from build123d import *

# Parameters (mm, degrees)
F0_R      = 1.6
F1_DEPTH  = 4.75
F2_W      = 25
F2_H      = 11
F3_DEPTH  = 12
F5_DEPTH  = 6
F7_DEPTH  = 5.5
F8_W      = 12
F8_H      = 11
F9_DEPTH  = 2
F10_W     = 12
F10_H     = 11
F11_DEPTH = 2
F12_R     = 1.45
F14_DEPTH = 25
F13_R     = 1.45
F15_DEPTH = 25
F16_R     = 5


with BuildPart() as f1:
    # F0 (on Front) → F1 (new body, symmetric)
    with BuildSketch(Plane.XZ):
        with BuildLine():
            ThreePointArc((35.398387, -3.5), (40.348135, 8.449747), (28.398387, 3.5))
            Line((28.398387, 3.5), (-35.398387, 3.5))
            ThreePointArc((-35.398387, 3.5), (-38.898387, 0), (-35.398387, -3.5))
            Line((-35.398387, -3.5), (35.398387, -3.5))
        make_face()
        with Locations((35.398387, 3.5)):
            Circle(F0_R, mode=Mode.SUBTRACT)
    extrude(amount=F1_DEPTH, both=True)

    # F2 (on face) → F3 (join)
    with BuildSketch(Plane(origin=(0, 4.75, 0), x_dir=(-1, 0, 0), z_dir=(0, 1, 0))):
        with Locations((0, 2)):
            Rectangle(F2_W, F2_H)
    extrude(amount=-F3_DEPTH)

    # F4 (on face) → F5 (cut)
    with BuildSketch(Plane.XY.offset(7.5)):
        with BuildLine():
            Line((-6, -7.25), (6, -7.25))
            ThreePointArc((6, -7.25), (0, -1.25), (-6, -7.25))
        make_face()
        with BuildLine():
            ThreePointArc((-6, -7.25), (0, -13.25), (6, -7.25))
            Line((6, -7.25), (-6, -7.25))
        make_face()
    extrude(amount=-F5_DEPTH, mode=Mode.SUBTRACT)

    # F6 (on face) → F7 (cut)
    with BuildSketch(Plane(origin=(0, 0, -3.5), x_dir=(1, 0, 0), z_dir=(0, 0, -1))):
        with BuildLine():
            Line((-8, 7.25), (8, 7.25))
            ThreePointArc((8, 7.25), (0, 15.25), (-8, 7.25))
        make_face()
        with BuildLine():
            ThreePointArc((-8, 7.25), (0, -0.75), (8, 7.25))
            Line((8, 7.25), (-8, 7.25))
        make_face()
    extrude(amount=-F7_DEPTH, mode=Mode.SUBTRACT)

    # F8 (on face) → F9 (join)
    with BuildSketch(Plane.YZ.offset(12.5)):
        with Locations((-1.25, 2)):
            Rectangle(F8_W, F8_H)
    extrude(amount=F9_DEPTH)

    # F10 (on face) → F11 (join)
    with BuildSketch(Plane(origin=(-12.5, 0, 0), x_dir=(0, -1, 0), z_dir=(-1, 0, 0))):
        with Locations((1.25, 2)):
            Rectangle(F10_W, F10_H)
    extrude(amount=F11_DEPTH)

    # F12 (on face) → F14 (cut)
    with BuildSketch(Plane.XZ.offset(7.25)):
        with Locations((-12.05, 3.05)):
            Circle(F12_R)
    extrude(amount=-F14_DEPTH, mode=Mode.SUBTRACT)

    # F13 (on face) → F15 (cut)
    with BuildSketch(Plane.XZ.offset(7.25)):
        with Locations((12.05, 3.05)):
            Circle(F13_R)
    extrude(amount=-F15_DEPTH, mode=Mode.SUBTRACT)

    # F16
    f16_edges = [f1.edges().sort_by_distance(p)[0] for p in [
        (-14.5, -6, -3.5),
        (-14.5, -1.25, 7.5),
        (14.5, -6, -3.5),
        (14.5, -1.25, 7.5),
    ]]
    fillet(f16_edges, radius=F16_R)


solid = f1.part
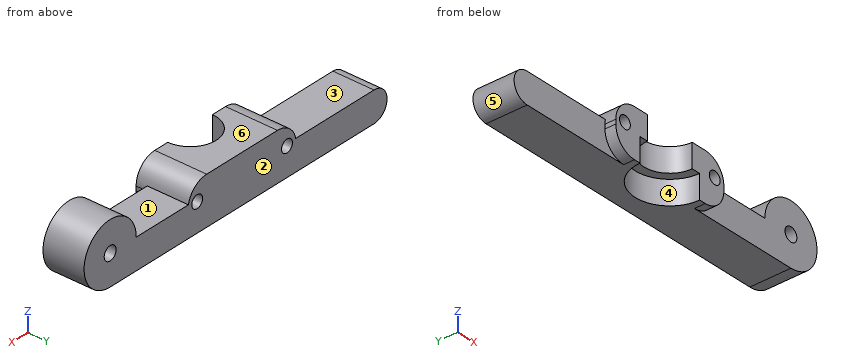
Check sheet for the modelled part. Datum: model origin and axes. Units: mm. Face numbers are marked on the shaded views. A direction names the side the tool comes from. Round coordinates to 2 decimals unless told otherwise and drop trailing zeros. Write each loop counter-clockwise with the first axis right and the second up, starting at its lowest first coordinate (ties: lowest second). Pieces come first, ordered by that corner, then holes. Notation, with made-up numbers: (-1.5, 80) -> (16.5, 80) arc R23 ccw to (16.5, 96) -> close; hole circle Ø6 at (88.25, 17). An arc over 180 degrees is marked (long way). Answer as CSV lines item,"result". Start each with the question number.
1) Material ranges on line 1 (X direction, y = -3, z = 3.75); line 2 (X direction, y = -3.75, z = 6.25); line 3 (Z direction, x = 9.5, y = 4), recorded low to high. Write a range as from..to.
2) Tool access check on the marked faces 1, 2 and 3. Record the directions out of +Z, -Z, +X, -X, +Y, -Y that give a thin tool (end or side, any length) a straight path to the whole face; none if there is none.
3) Section check D-D on x = 32. Enter the section's corners in (y, z).
4) Section check C-C on x = 0. Enter the section's corners in (y, z), and give its area (3 significant figures).
5) Section check B-B on z = 0. Enter the section's corners in (x, y).
6) Release check for a two-part mould opening along X. For the marked faces 4, 5 and 6 record: pulls with the +X half, pulls with the -X half, needs draft (parallel to the pull), parting line crosses it, or undercut.
7) Section check A-A on x = 12.05. Enter the section's corners in (y, z), and give its area (3 significant figures).
8) Go/stop test with flat-tipped pins: P1, Ø7.5, axis at x = -28.5, z = -0.5, coming from the -Y side; P2, Ø4, axis at x = -1, z = 0.5, coming from the -Y side; P3, Ø0.5, axis at y = -6, z = 2, coming from the +X side. Record where each tip stops, or that it passes through.
Found:
1,line 1,"x = -14.34..-13.32, -10.78..-4.24, 4.24..10.78, 13.32..14.34, 28.4..33.82, 36.98..42.39"
1,line 2,"x = -12.81..-4.87, 4.87..12.81, 28.96..41.84"
1,line 3,"z = -3.5..7.5"
2,face 1,"+Z, +Y, -Y"
2,face 2,"+Z, -Z, +X, -X, +Y"
2,face 3,"+Z, -X, +Y, -Y"
3,outline,"(-4.75, -3.5) -> (4.75, -3.5) -> (4.75, 9.62) -> (-4.75, 9.62) -> close"
4,outline,"(-1.25, 2) -> (0.75, 2) -> (0.75, -3.5) -> (4.75, -3.5) -> (4.75, 7.5) -> (-1.25, 7.5) -> close"
4,area,"55.0 mm^2"
5,outline,"(-38.9, -4.75) -> (-14.27, -4.75) -> (-14.27, -7.25) -> (-8, -7.25) arc R8 cw to (8, -7.25) -> (14.27, -7.25) -> (14.27, -4.75) -> (41.46, -4.75) -> (41.46, 4.75) -> (-38.9, 4.75) -> close"
6,face 4,"undercut"
6,face 5,"pulls with the -X half"
6,face 6,"needs draft"
7,outline,"(-7.25, -2.8) -> (-4.75, -2.8) -> (-4.75, -3.5) -> (4.75, -3.5) -> (4.75, 1.6) -> (-7.25, 1.6) -> close; (-7.25, 4.5) -> (4.75, 4.5) -> (4.75, 6.8) -> (-7.25, 6.8) -> close"
7,area,"87.1 mm^2"
8,P1,"stops at y = -4.75"
8,P2,"stops at y = -1.72"
8,P3,"stops at x = 14.5"
